from build123d import *

# Parameters (mm, degrees)
SKETCH_1_W                      = 4
SKETCH_1_H                      = 49.98
LEFT_RF_PLATE_DEPTH             = 8.851909566
SKETCH_2_R                      = 0.8
FRAME_2XD1P6_THROUGH_DEPTH      = 47.728029093
SKETCH_3_R                      = 2.05
SMA_CENTER_D4P1_DEPTH           = 4
SKETCH_4_R                      = 0.875
SMA_UPPER_2XD1P75_THROUGH_DEPTH = 48.179152176


with BuildPart() as part:
    # 草图1 → Left_RF_Plate (new body)
    with BuildSketch(Plane.XY):
        with Locations((-2.3, 20.69)):
            Rectangle(SKETCH_1_W, SKETCH_1_H)
    extrude(amount=LEFT_RF_PLATE_DEPTH)


with BuildPart() as part_1:
    # Stock_Z_Position: moved
    add(part.part.moved(Location((0, 0, 2.248090434))))

    # 草图2 → Frame_2xD1p6_Through (cut, through all)
    with BuildSketch(Plane.XY.offset(11.1)):
        with Locations((-2.3, -1)):
            Circle(SKETCH_2_R)
        with Locations((-2.3, 43)):
            Circle(SKETCH_2_R)
    extrude(amount=-FRAME_2XD1P6_THROUGH_DEPTH, mode=Mode.SUBTRACT)

    # 草图3 → SMA_Center_D4p1 (cut)
    with BuildSketch(Plane.ZY.offset(4.3)):
        with Locations((3.899496327, 10.725)):
            Circle(SKETCH_3_R)
    extrude(amount=-SMA_CENTER_D4P1_DEPTH, mode=Mode.SUBTRACT)

    # 草图4 → SMA_Upper_2xD1p75_Through (cut, through all)
    with BuildSketch(Plane.ZY.offset(4.3)):
        with Locations((8.199496327, 6.425)):
            Circle(SKETCH_4_R)
        with Locations((8.199496327, 15.025)):
            Circle(SKETCH_4_R)
    extrude(amount=-SMA_UPPER_2XD1P75_THROUGH_DEPTH, mode=Mode.SUBTRACT)


solid = part_1.part
Work out the finished part from the listing and answer in its coordinate system (mm). Round coordinates to 2 decimals unless told otherwise and drop trailing zeros. Write each loop counter-clockwise with the first axis right and the second up, starting at its lowest first coordinate (ties: lowest second). Pieces come first, ordered by that corner, then holes. Notation, with made-up numbers: (-30, -25) -> (5, -25) arc R28 ccw to (5, 4) -> close; hole circle Ø4 at (-23, 8.25). An arc over 180 degrees is marked (long way). Answer as CSV lines item,"result". Start each with the question number.
(1) The part is cut by section A-A, the plane y = -1. Give the vertices of the cut face in (x, z).
(2) The mould has two halves that part along X. Classify faces 1 (the flat face through (-4.3, 20, 7)), 2 (the cylindrical face through (-2.33, 10.65, 5.95)), 3 (the cylindrical face through (-3.1, -1, 6.7)), 4 (the cylindrical face through (-2.404, 43.793, 6.736)): +X half, -X half, draft (parallel to the pull), parting line (faces both ways), or undercut.
(3) Find the intervals of material crossed by probe 1 along Y at (x, z) = (-2.25, 4); probe 2 along Y at (x, z) = (-2.3, 4.5); probe 3 along X at (y, z) = (43, 8.25), in increasing order.
(4) The part is cut by section D-D, the plane z = 3. Give the vertices of the cut face in (x, y), then the cut area to 3 significant figures.
(5) The part is cut by section B-B, the plane z = 8. Give the vertices of the cut face in (x, y), then the cut area to 3 significant figures.
(6) The part is cut by section C-C, the plane x = -2.3. Give the number of separate pieces and of enclosed holes in the cut face, then the cut area to 3 significant figures.
Output values:
1,outline,"(-4.3, 2.25) -> (-3.1, 2.25) -> (-3.1, 11.1) -> (-4.3, 11.1) -> close; (-1.5, 2.25) -> (-0.3, 2.25) -> (-0.3, 11.1) -> (-1.5, 11.1) -> close"
2,face 1,"-X half"
2,face 2,"draft"
2,face 3,"undercut"
2,face 4,"undercut"
3,probe 1,"y = -4.3 to -1.8, -0.2 to 8.68, 12.77 to 42.2, 43.8 to 45.68"
3,probe 2,"y = -4.3 to -1.8, -0.2 to 8.76, 12.69 to 42.2, 43.8 to 45.68"
3,probe 3,"x = -4.3 to -3.1, -1.5 to -0.3"
4,outline,"(-4.3, -4.3) -> (-0.3, -4.3) -> (-0.3, 8.88) -> (-4.3, 8.88) -> close; (-4.3, 12.57) -> (-0.3, 12.57) -> (-0.3, 45.68) -> (-4.3, 45.68) -> close; hole circle Ø1.6 at (-2.3, -1); hole circle Ø1.6 at (-2.3, 43)"
4,area,"181 mm²"
5,outline,"(-4.3, -4.3) -> (-0.3, -4.3) -> (-0.3, 5.57) -> (-4.3, 5.57) -> close; (-4.3, 7.28) -> (-0.3, 7.28) -> (-0.3, 14.17) -> (-4.3, 14.17) -> close; (-4.3, 15.88) -> (-0.3, 15.88) -> (-0.3, 45.68) -> (-4.3, 45.68) -> close; hole circle Ø1.6 at (-2.3, -1); hole circle Ø1.6 at (-2.3, 43)"
5,area,"182 mm²"
6,separate pieces,"3"
6,enclosed holes,"2"
6,area,"397 mm²"
